Verification items for the finished model (mm, model axes). Face numbers are marked on the shaded views. A direction names the side the tool comes from. Round coordinates to 2 decimals unless told otherwise and drop trailing zeros. Write each loop counter-clockwise with the first axis right and the second up, starting at its lowest first coordinate (ties: lowest second). Pieces come first, ordered by that corner, then holes.
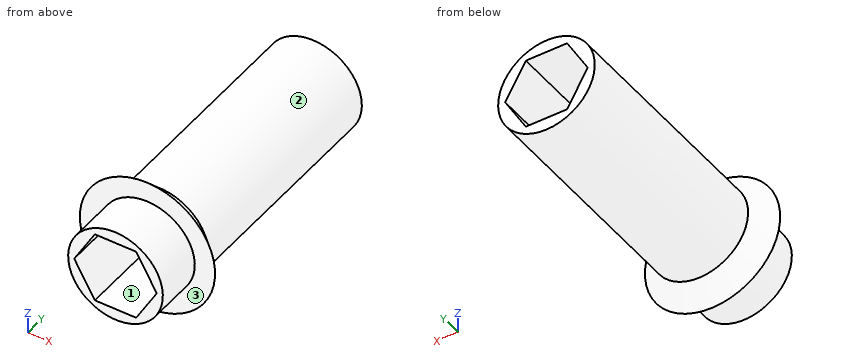
from build123d import *

# Parameters (mm, degrees)
SKETCH_1_R      = 4.9
EXTRUDE_1_DEPTH = 5
SKETCH_2_R      = 5
EXTRUDE_2_DEPTH = 26
SKETCH_5_R      = 7
SKETCH_5_R_2    = 5
EXTRUDE_4_DEPTH = 2
CHAMFER_1_SIZE  = 2


with BuildPart() as part:
    # 草图1 → 凸台-拉伸1 (new body)
    with BuildSketch(Plane(origin=(0, 0, 0), x_dir=(1, 0, 0), z_dir=(0, 1, 0))):
        with Locations(Location((0, 0, 0), (0, 0, 270))):
            Circle(SKETCH_1_R)
        Polygon((4.272391992, 0), (2.136195996, 3.7), (-2.136195996, 3.7), (-4.272391992, 0), (-2.136195996, -3.7), (2.136195996, -3.7), align=None, mode=Mode.SUBTRACT)
    extrude(amount=EXTRUDE_1_DEPTH)

    # 草图2 → 凸台-拉伸2 (add)
    with BuildSketch(Plane(origin=(0, 5, 0), x_dir=(1, 0, 0), z_dir=(0, 1, 0))):
        with Locations(Location((0, 0, 0), (0, 0, 90))):
            Circle(SKETCH_2_R)
        Polygon((4.272391992, 0), (2.136195996, 3.7), (-2.136195996, 3.7), (-4.272391992, 0), (-2.136195996, -3.7), (2.136195996, -3.7), align=None, mode=Mode.SUBTRACT)
    extrude(amount=EXTRUDE_2_DEPTH)

    # 草图5 → 凸台-拉伸4 (add)
    with BuildSketch(Plane.XZ.offset(-5)):
        with Locations(Location((0, 0, 0), (0, 0, 270))):
            Circle(SKETCH_5_R)
        with Locations(Location((0, 0, 0), (0, 0, 270))):
            Circle(SKETCH_5_R_2, mode=Mode.SUBTRACT)
    extrude(amount=-EXTRUDE_4_DEPTH)

    # 倒角1
    chamfer_1_edges = [part.edges().sort_by_distance(p)[0] for p in [
        (0, 7, 7),
    ]]
    chamfer(chamfer_1_edges, length=CHAMFER_1_SIZE - 0.0001)  # a hair under: the kernel refuses the full size


solid = part.part
Q1. Depth check by flat-ended pin: P1, Ø1.3, axis at x = 0.5, y = 10.5, coming from the -Z side; P2, Ø5, axis at y = 19.5, z = 2.5, coming from the +X side; P3, Ø1.5, axis at x = 2, z = -1.5, coming from the -Y side; P4, Ø1, axis at x = 5, z = -4.5, coming from the -Y side. Enter the tip coordinate at first touch or a pass-through.
Recorded:
P1: stops at z = -5
P2: stops at x = 5
P3: passes through
P4: stops at y = 5
Q2. Material ranges on line 1 along X through (y, z) = (28, -3); line 2 along X through (y, z) = (16, -3.5); line 3 along Z through (x, y) = (-2.5, 3.5), recorded low to high.
Recorded:
line 1: x = -4 to -2.54, 2.54 to 4
line 2: x = -3.57 to -2.25, 2.25 to 3.57
line 3: z = -4.21 to -3.07, 3.07 to 4.21
Q3. Tool access check on the marked faces 1, 2 and 3. Record the directions out of +Z, -Z, +X, -X, +Y, -Y that give a thin tool (end or side, any length) a straight path to the whole face; none if there is none.
Recorded:
face 1: +Y, -Y
face 2: +Y
face 3: -Y
Q4. Sectioned sample at B-B (y = 22). Enter the section's corners in (x, z).
Recorded:
outline: circle Ø10 at (0, 0); hole (-4.27, 0) - (-2.14, -3.7) - (2.14, -3.7) - (4.27, 0) - (2.14, 3.7) - (-2.14, 3.7) - close
